Build history of the part. All positions in model axes, mm. A direction names the side the tool comes from. Give positions to 0.01 mm unless a question says otherwise; leave off trailing zeros. Order: outer loops, then holes, each group sorted by start corner. A loop starts at its lowest first (then second) coordinate and runs counter-clockwise, first axis right, second up. Notation, with made-up numbers: M 49,33.5 L 103,33.5 A35 cw 103,68.5 Z; hole C 33.5,65 d10. An arc over 180 degrees is marked long. One line per item, written item: value. Start each with the question number.
from build123d import *

# Parameters (mm, degrees)
RESSALTO_EXTRUS_O1_DEPTH      = 65
RESSALTO_EXTRUS_O1_DEPTH_BACK = 30
ESBO_O1_R                     = 2
CORTE_EXTRUS_O4_DEPTH         = 25.015
CORTE_EXTRUS_O5_DEPTH         = 55.015


with BuildPart() as part:
    # Esboço1 → Ressalto-extrusão1 (new, two sides: drawn at the far end of the back side and taken through both)
    with BuildSketch(Plane.XY.offset(-RESSALTO_EXTRUS_O1_DEPTH_BACK)):
        Circle(ESBO_O1_R)
    extrude(amount=RESSALTO_EXTRUS_O1_DEPTH + RESSALTO_EXTRUS_O1_DEPTH_BACK)

    # Esboço5 → Corte-extrusão4 (cut)
    with BuildSketch(Plane.XY.offset(65)):
        Polygon((0, 1.425), (2.691542187, 1.425), (2.691542187, 2.754428638), (-3.67257147, 2.754428638), (-3.67257147, 1.425), align=None)
        Polygon((0, -1.425), (2.691542187, -1.425), (2.691542187, -2.855047036), (-3.67257147, -2.855047036), (-3.67257147, -1.425), align=None)
    extrude(amount=-CORTE_EXTRUS_O4_DEPTH, mode=Mode.SUBTRACT)

    # Esboço6 → Corte-extrusão5 (cut)
    with BuildSketch(Plane(origin=(0, 0, -30), x_dir=(-1, 0, 0), z_dir=(0, 0, -1))):
        Polygon((0, 1.425), (2.641232941, 1.425), (2.641232941, 2.588827525), (-2.871816769, 2.588827525), (-2.871816769, 1.425), align=None)
        Polygon((0, -1.425), (2.641232941, -1.425), (2.641232941, -2.693638356), (-2.871816769, -2.693638356), (-2.871816769, -1.425), align=None)
    extrude(amount=-CORTE_EXTRUS_O5_DEPTH, mode=Mode.SUBTRACT)


solid = part.part
1) Drop flat-ended pins along their axis: P1, Ø1.4, axis at x = 0, z = -7, coming from the +Y side (3 decimals); P2, Ø0.6, axis at x = 0.5, y = 2, coming from the -Z side (3 decimals); P3, Ø0.6, axis at x = 0, y = -2, coming from the +Z side (3 decimals); P4, Ø0.5, axis at x = 0, y = 1.5, coming from the +Z side. Give the stop position or say it passes through.
2) Drill centre lines: line 1 (Y direction, x = -0.4, z = 43.5) (3 decimals); line 2 (X direction, y = -0.15, z = 35); line 3 (X direction, y = -1, z = 27.5). Where is each one in solid material? Low to high.
3) Slice it at A-A (x = 0). List the corners of the cut face in (y, z) (3 decimals), plus the area to 3 significant figures.
4) Slice it at B-B (z = 33.5). List the corners of the cut face in (x, y), plus the area to 3 significant figures.
5) Slice it at C-C (z = 49.5). List the corners of the cut face in (x, y) (3 decimals).
6) Tool access for faces 1 (the flat face through (0, 1.425, 53)), 2 (the flat face through (0, -1.425, 53)), 3 (the flat face through (0, -1.425, -3)), 4 (the flat face through (0, 1.425, -3)): list every direction of +Z, -Z, +X, -X, +Y, -Y with a clear straight run to the whole face (end or side of a thin tool).
Results list:
1. P1: stops at y = 1.425
1. P2: stops at z = 25.015
1. P3: stops at z = 39.985
1. P4: stops at z = 65
2. line 1: y = -1.425 to 1.425
2. line 2: x = -1.99 to 1.99
2. line 3: x = -1.73 to 1.73
3. outline: M -2,25.015 L -1.425,25.015 L -1.425,-30 L 1.425,-30 L 1.425,25.015 L 2,25.015 L 2,39.985 L 1.425,39.985 L 1.425,65 L -1.425,65 L -1.425,39.985 L -2,39.985 Z
3. area: 288 mm²
4. outline: C 0,0 d4
4. area: 12.6 mm²
5. outline: M -1.403,-1.425 L 1.403,-1.425 A2 ccw 1.403,1.425 L -1.403,1.425 A2 ccw Z
6. face 1: +Z, +X, -X, +Y
6. face 2: +Z, +X, -X, -Y
6. face 3: -Z, +X, -X, -Y
6. face 4: -Z, +X, -X, +Y
